```python
from build123d import *

# Parameters (mm, degrees)
BOSS_EXTRUDE1_DEPTH             = 5
BOSS_EXTRUDE2_REACH             = 185.439
SKETCH2_R                       = 1.25
BOSS_EXTRUDE2_DIRECTION_2_REACH = 185.439
CUT_EXTRUDE1_DEPTH              = 188.472664674
CUT_EXTRUDE1_DEPTH_BACK         = 188.472664674
SKETCH4_W                       = 14.3
SKETCH4_H                       = 48.6
SKETCH5_RX                      = 1.25
SKETCH5_RY                      = 0.173611111
SKETCH5_R                       = 16.2
BOSS_EXTRUDE3_DEPTH             = 16.5
SKETCH7_R                       = 16.2
SKETCH7_R_2                     = 14.7
BOSS_EXTRUDE5_DEPTH             = 0.5
CUT_EXTRUDE2_DEPTH              = 190.224443453
FILLET2_R                       = 2
FILLET5_R                       = 2
CHAMFER1_SIZE                   = 0.5
FILLET6_R                       = 2


with BuildPart() as part:
    # Sketch1 → Boss-Extrude1 (new body)
    with BuildSketch(Plane(origin=(0, 0, 0), x_dir=(1, 0, 0), z_dir=(0, 1, 0))):
        Polygon((0, -35), (0, 35), (180, 10), (180, -10), align=None)
    extrude(amount=BOSS_EXTRUDE1_DEPTH)

    # Boss-Extrude2: up to this plane
    boss_extrude2_end = Plane(origin=(4.769114307, 5, 34.337623013), z_dir=(-0.1375683712746877, 0, -0.9904922731777516))
    # Sketch2 → Boss-Extrude2 (add, up to the surface)
    with BuildSketch(Plane.XY, mode=Mode.PRIVATE) as boss_extrude2_sk1:
        with BuildLine():
            Line((0, 33), (0, 5))
            Line((0, 5), (12, 5))
            Line((12, 5), (12, 33))
            ThreePointArc((12, 33), (6, 39), (0, 33))
        make_face()
        Polygon((2.5, 8), (6, 16), (9.5, 8), align=None, mode=Mode.SUBTRACT)
        Polygon((2.5, 12.989785485), (2.5, 21.010214515), (4.25446885, 17), align=None, mode=Mode.SUBTRACT)
        Polygon((7.74553115, 17), (9.5, 21.010214515), (9.5, 12.989785485), align=None, mode=Mode.SUBTRACT)
        Polygon((6, 18), (2.5, 26), (9.5, 26), align=None, mode=Mode.SUBTRACT)
        with Locations((6, 33)):
            Circle(SKETCH2_R, mode=Mode.SUBTRACT)
    boss_extrude2_tool1 = split(extrude(boss_extrude2_sk1.sketch, amount=BOSS_EXTRUDE2_REACH, mode=Mode.PRIVATE), bisect_by=boss_extrude2_end, keep=Keep.BOTH, mode=Mode.PRIVATE)
    add(boss_extrude2_tool1.solids().sort_by_distance((11.639445, 19, 0))[0])
    # Sketch2 → Boss-Extrude2 (add, up to the surface)
    with BuildSketch(Plane.XY, mode=Mode.PRIVATE) as boss_extrude2_sk2:
        with BuildLine():
            Line((168, 8), (168, 5))
            Line((168, 5), (180, 5))
            Line((180, 5), (180, 8))
            ThreePointArc((180, 8), (174, 14), (168, 8))
        make_face()
        with Locations((174, 8)):
            Circle(SKETCH2_R, mode=Mode.SUBTRACT)
    boss_extrude2_tool2 = split(extrude(boss_extrude2_sk2.sketch, amount=BOSS_EXTRUDE2_REACH, mode=Mode.PRIVATE), bisect_by=boss_extrude2_end, keep=Keep.BOTH, mode=Mode.PRIVATE)
    add(boss_extrude2_tool2.solids().sort_by_distance((168.15, 6.5, 0))[0])

    # Boss-Extrude2 direction 2: up to this plane
    boss_extrude2_direction_2_end = Plane(origin=(4.769114307, 5, -34.337623013), z_dir=(-0.1375683712746877, 0, 0.9904922731777516))
    # Sketch2 → Boss-Extrude2 direction 2 (add, up to the surface)
    with BuildSketch(Plane.XY, mode=Mode.PRIVATE) as boss_extrude2_direction_2_sk1:
        with BuildLine():
            Line((0, 33), (0, 5))
            Line((0, 5), (12, 5))
            Line((12, 5), (12, 33))
            ThreePointArc((12, 33), (6, 39), (0, 33))
        make_face()
        Polygon((2.5, 8), (6, 16), (9.5, 8), align=None, mode=Mode.SUBTRACT)
        Polygon((2.5, 12.989785485), (2.5, 21.010214515), (4.25446885, 17), align=None, mode=Mode.SUBTRACT)
        Polygon((7.74553115, 17), (9.5, 21.010214515), (9.5, 12.989785485), align=None, mode=Mode.SUBTRACT)
        Polygon((6, 18), (2.5, 26), (9.5, 26), align=None, mode=Mode.SUBTRACT)
        with Locations((6, 33)):
            Circle(SKETCH2_R, mode=Mode.SUBTRACT)
    boss_extrude2_direction_2_tool1 = split(extrude(boss_extrude2_direction_2_sk1.sketch, amount=-BOSS_EXTRUDE2_DIRECTION_2_REACH, mode=Mode.PRIVATE), bisect_by=boss_extrude2_direction_2_end, keep=Keep.BOTH, mode=Mode.PRIVATE)
    add(boss_extrude2_direction_2_tool1.solids().sort_by_distance((11.639445, 19, 0))[0])
    # Sketch2 → Boss-Extrude2 direction 2 (add, up to the surface)
    with BuildSketch(Plane.XY, mode=Mode.PRIVATE) as boss_extrude2_direction_2_sk2:
        with BuildLine():
            Line((168, 8), (168, 5))
            Line((168, 5), (180, 5))
            Line((180, 5), (180, 8))
            ThreePointArc((180, 8), (174, 14), (168, 8))
        make_face()
        with Locations((174, 8)):
            Circle(SKETCH2_R, mode=Mode.SUBTRACT)
    boss_extrude2_direction_2_tool2 = split(extrude(boss_extrude2_direction_2_sk2.sketch, amount=-BOSS_EXTRUDE2_DIRECTION_2_REACH, mode=Mode.PRIVATE), bisect_by=boss_extrude2_direction_2_end, keep=Keep.BOTH, mode=Mode.PRIVATE)
    add(boss_extrude2_direction_2_tool2.solids().sort_by_distance((168.15, 6.5, 0))[0])

    # Sketch4 → Cut-Extrude1 (cut, two sides: drawn at the far end of the back side and taken through both)
    with BuildSketch(Plane(origin=(0, 0, 0), x_dir=(1, 0, 0), z_dir=(0, 1, 0)).offset(-CUT_EXTRUDE1_DEPTH_BACK)):
        with Locations((7.15, 0)):
            Rectangle(SKETCH4_W, SKETCH4_H)
    extrude(amount=CUT_EXTRUDE1_DEPTH + CUT_EXTRUDE1_DEPTH_BACK, mode=Mode.SUBTRACT)

    # Sketch5 → Boss-Extrude3 (add)
    # profile 1 of 2: a face of its own
    with BuildSketch(Plane.ZY.offset(-14.3)):
        with Locations(Location((-34.166666667, 33), (0, 0, 90))):
            Ellipse(SKETCH5_RX, SKETCH5_RY)
    # profile 2 of 2: a face of its own
    with BuildSketch(Plane.ZY.offset(-14.3)):
        with BuildLine():
            Line((-18.7, 5), (-18.7, 33))
            ThreePointArc((-18.7, 33), (0, 51.7), (18.7, 33))
            Line((18.7, 33), (18.7, 5))
            Line((18.7, 5), (-18.7, 5))
        make_face()
        with Locations((0, 33)):
            Circle(SKETCH5_R, mode=Mode.SUBTRACT)
        with BuildLine():
            Line((16.2, 7.5), (16.2, 14.173334694))
            ThreePointArc((16.2, 14.173334694), (9.90483685, 9.7420086), (2.5, 7.63627327))
            Line((2.5, 7.63627327), (2.5, 7.5))
            Line((2.5, 7.5), (16.2, 7.5))
        make_face(mode=Mode.SUBTRACT)
        with BuildLine():
            Line((-16.2, 7.5), (-16.2, 14.173334694))
            ThreePointArc((-16.2, 14.173334694), (-9.90483685, 9.7420086), (-2.5, 7.63627327))
            Line((-2.5, 7.63627327), (-2.5, 7.5))
            Line((-2.5, 7.5), (-16.2, 7.5))
        make_face(mode=Mode.SUBTRACT)
    extrude(amount=-BOSS_EXTRUDE3_DEPTH)


with BuildPart() as boss_extrude3_kept_piece:
    # of the separate pieces the step leaves, the one the design keeps (boss_extrude3_pieces_kept)
    add(part.part.solids().sort_by_distance((0, 0, 35))[0])

    # Sketch7 → Boss-Extrude5 (add, symmetric)
    # profile 1 of 2: a face of its own
    with BuildSketch(Plane(origin=(30.8, 0, 0), x_dir=(0, 0, -1), z_dir=(1, 0, 0))):
        with BuildLine():
            Line((18.7, 5), (18.7, 33))
            ThreePointArc((18.7, 33), (0, 51.7), (-18.7, 33))
            Line((-18.7, 33), (-18.7, 5))
            Line((-18.7, 5), (18.7, 5))
        make_face()
        with Locations(Location((0, 33, 0), (0, 0, 180))):
            Circle(SKETCH7_R, mode=Mode.SUBTRACT)
        with BuildLine():
            ThreePointArc((-16.2, 14.173334694), (-9.90483685, 9.7420086), (-2.5, 7.63627327))
            Line((-2.5, 7.63627327), (-2.5, 7.5))
            Line((-2.5, 7.5), (-16.2, 7.5))
            Line((-16.2, 7.5), (-16.2, 14.173334694))
        make_face(mode=Mode.SUBTRACT)
        with BuildLine():
            ThreePointArc((2.5, 7.63627327), (9.90483685, 9.7420086), (16.2, 14.173334694))
            Line((16.2, 14.173334694), (16.2, 7.5))
            Line((16.2, 7.5), (2.5, 7.5))
            Line((2.5, 7.5), (2.5, 7.63627327))
        make_face(mode=Mode.SUBTRACT)
    # profile 2 of 2: a face of its own
    with BuildSketch(Plane(origin=(30.8, 0, 0), x_dir=(0, 0, -1), z_dir=(1, 0, 0))):
        with Locations(Location((0, 33, 0), (0, 0, 180))):
            Circle(SKETCH7_R)
        with Locations((0, 33)):
            Circle(SKETCH7_R_2, mode=Mode.SUBTRACT)
    extrude(amount=BOSS_EXTRUDE5_DEPTH, both=True)

    # Sketch8 → Cut-Extrude2 (cut, through all)
    with BuildSketch(Plane(origin=(0, 5, 0), x_dir=(1, 0, 0), z_dir=(0, 1, 0))):
        Polygon((40, 17.5), (40, -17.5), (160, 0), align=None)
    extrude(amount=-CUT_EXTRUDE2_DEPTH, mode=Mode.SUBTRACT)

    # Fillet2
    fillet2_edges = [boss_extrude3_kept_piece.edges().sort_by_distance(p)[0] for p in [
        (40, 2.5, -17.5),
        (160, 2.5, 0),
        (40, 2.5, 17.5),
    ]]
    fillet(fillet2_edges, radius=FILLET2_R)

    # Fillet5
    fillet5_edges = [boss_extrude3_kept_piece.edges().sort_by_distance(p)[0] for p in [
        (14.3, 2.5, 24.3),
        (14.3, 2.5, -24.3),
    ]]
    fillet(fillet5_edges, radius=FILLET5_R)

    # Chamfer1
    chamfer1_edges = [boss_extrude3_kept_piece.edges().sort_by_distance(p)[0] for p in [
        (14.3, 33, -16.2),
    ]]
    chamfer(chamfer1_edges, length=CHAMFER1_SIZE)

    # Fillet6
    fillet6_edges = [boss_extrude3_kept_piece.edges().sort_by_distance(p)[0] for p in [
        (12, 19, 33.333333333),
        (6, 39, -34.166666667),
        (6, 39, 34.166666667),
        (12, 19, -33.333333333),
        (174, 14, -10.833333333),
        (168, 6.5, -11.666666667),
        (174, 14, 10.833333333),
        (168, 6.5, 11.666666667),
        (180, 4, 10),
        (0, 16.5, 35),
        (0, 16.5, -35),
        (180, 4, -10),
    ]]
    fillet(fillet6_edges, radius=FILLET6_R)


solid = boss_extrude3_kept_piece.part
```
Design review of the part built by this model. Coordinates are the model's own, in mm. A direction names the side the tool comes from. Round coordinates to 2 decimals unless told otherwise and drop trailing zeros. Write each loop counter-clockwise with the first axis right and the second up, starting at its lowest first coordinate (ties: lowest second). Pieces come first, ordered by that corner, then holes. Notation, with made-up numbers: (87, -11.5) -> (125, -11.5) arc R20 cw to (125, 11.5) -> close; hole circle Ø1 at (-35, -31.75). An arc over 180 degrees is marked (long way). Answer in a Markdown table with one row per item.
Q1. Take a section at A-A, the plane z = 0. State the section outline as (x, y) points, then the cut area to 3 significant figures.
The answers:
| item | result |
|---|---|
| outline | (14.3, 0) -> (40, 0) -> (40, 5) -> (31.3, 5) -> (31.3, 18.3) -> (30.3, 18.3) -> (30.3, 16.8) -> (14.8, 16.8) -> (14.3, 16.3) -> close; (14.3, 49.7) -> (14.8, 49.2) -> (30.3, 49.2) -> (30.3, 47.7) -> (31.3, 47.7) -> (31.3, 51.7) -> (14.3, 51.7) -> close; (148.14, 0) -> (180, 0) -> (180, 8) arc R6 ccw to (168, 8) -> (168, 5) -> (148.14, 5) -> close; hole circle Ø2.5 at (174, 8) |
| area | 621 mm² |
Q2. Take a section at B-B, the plane x = 54.5. State the section outline as (y, z) points.
The answers:
| item | result |
|---|---|
| outline | (0, -27.43) -> (5, -27.43) -> (5, -15.39) -> (0, -15.39) -> close; (0, 15.39) -> (5, 15.39) -> (5, 27.43) -> (0, 27.43) -> close |
Q3. Take a section at D-D, the plane x = 28. State the section outline as (y, z) points.
The answers:
| item | result |
|---|---|
| outline | (0, -31.11) -> (5, -31.11) -> (5, -18.7) -> (33, -18.7) arc R18.7 ccw to (33, 18.7) -> (5, 18.7) -> (5, 31.11) -> (0, 31.11) -> close; hole (7.5, -16.2) -> (14.17, -16.2) arc R23 cw to (7.64, -2.5) -> (7.5, -2.5) -> close; hole (7.5, 2.5) -> (7.64, 2.5) arc R23 cw to (14.17, 16.2) -> (7.5, 16.2) -> close; hole circle Ø32.4 at (33, 0) |
Q4. Clearance check with flat-ended pins moving along their axes: pin 1 Ø3.5 at (x, z) = (6.5, -27.5) entering from -Y; pin 2 Ø8 at (x, z) = (19.5, -26) entering from +Y; pin 3 Ø3.5 at (y, z) = (19.5, 28.5) entering from +X; pin 4 Ø5 at (y, z) = (23.5, 9.5) entering from +X. State where each tip first meets the part, or that it passes through.
The answers:
| item | result |
|---|---|
| pin 1 | y = 0 |
| pin 2 | y = 5 |
| pin 3 | x = 12 |
| pin 4 | x = 31.3 |
Q5. Draft analysis for pull direction Z (two halves, no side actions). For faces 4 (the face through (23, 19, 18.7)), 5 (the face through (22.681, 9.789, 10.002)), 6 (the face through (23, 7.5, -9)), 7 (the face through (6, 8, -29)), state which applies: +Z half, -Z half, draft (parallel to the pull), parting line (faces both ways), or undercut.
The answers:
| item | result |
|---|---|
| face 4 | +Z half |
| face 5 | undercut |
| face 6 | undercut |
| face 7 | draft |
Q6. Take a section at C-C, the plane z = 28.5. State the section outline as (x, y) points.
The answers:
| item | result |
|---|---|
| outline | (0, 0) -> (46.8, 0) -> (46.8, 5) -> (12, 5) -> (12, 33) arc R6 ccw to (0, 33) -> close; hole (2.5, 8) -> (9.5, 8) -> (6, 16) -> close; hole (2.5, 12.99) -> (4.25, 17) -> (2.5, 21.01) -> close; hole (2.5, 26) -> (6, 18) -> (9.5, 26) -> close; hole circle Ø2.5 at (6, 33); hole (7.75, 17) -> (9.5, 12.99) -> (9.5, 21.01) -> close |
Q7. To check wall thickness, follow L1, parallel to X at y = 33, z = -29.25; L2, parallel to Z at x = 23, y = 33; L3, parallel to X at y = 8, z = -1. State the ranges of each line that lie inside material, in increasing order. Write a range as [from, to].
The answers:
| item | result |
|---|---|
| L1 | [0, 4.75], [7.25, 12] |
| L2 | [-18.7, -16.2], [16.2, 18.7] |
| L3 | [14.3, 31.3], [168, 172.75], [175.25, 180] |
Q8. For faces 1 (the face through (14.3, 12, 0)), 2 (the face through (6, 26, -29)), 3 (the face through (23, 7.5, 9)), list the 3-axis set-ups (+Z, -Z, +X, -X, +Y, -Y) from which the entire face can be reached by the end or side of a thin tool; tool diameter is ignored.
The answers:
| item | result |
|---|---|
| face 1 | -X, +Y, -Y |
| face 2 | +Z, -Z |
| face 3 | -X |
